```python
from build123d import *

# Parameters (mm, degrees)
SKETCH1_W               = 1500
SKETCH1_H               = 500
BOSS_EXTRUDE1_DEPTH     = 80
FILLET2_R               = 10
CUT_EXTRUDE2_START      = 80
SKETCH7_W               = 720
SKETCH7_H               = 439.016917436
CUT_EXTRUDE2_DEPTH      = 2
CUT_EXTRUDE1_START      = 78
SKETCH5_W               = 66
SKETCH5_H               = 45
CUT_EXTRUDE1_DEPTH      = 10
CUT_EXTRUDE3_START      = 80
SKETCH8_R               = 5
CUT_EXTRUDE3_DEPTH      = 875.606821013
CUT_EXTRUDE4_DEPTH      = 100
CUT_EXTRUDE4_DEPTH_BACK = 100
SKETCH9_W               = 720
SKETCH9_H               = 40
SKETCH11_R              = 10
CUT_EXTRUDE5_DEPTH      = 250


with BuildPart() as part:
    # Sketch1 → Boss-Extrude1 (new body)
    with BuildSketch(Plane(origin=(0, 0, 0), x_dir=(1, 0, 0), z_dir=(0, 1, 0))):
        Rectangle(SKETCH1_W, SKETCH1_H)
    extrude(amount=BOSS_EXTRUDE1_DEPTH)

    # Fillet2
    fillet2_edges = [part.edges().sort_by_distance(p)[0] for p in [
        (-750, 80, 0),
        (0, 80, 250),
        (750, 80, 0),
        (0, 80, -250),
    ]]
    fillet(fillet2_edges, radius=FILLET2_R)

    # Sketch7 → Cut-Extrude2 (cut)
    with BuildSketch(Plane(origin=(0, 0, 0), x_dir=(1, 0, 0), z_dir=(0, 1, 0)).offset(CUT_EXTRUDE2_START)):
        with Locations((0, 157.008458718)):
            Rectangle(SKETCH7_W, SKETCH7_H)
    extrude(amount=-CUT_EXTRUDE2_DEPTH, mode=Mode.SUBTRACT)

    # Sketch5 → Cut-Extrude1 (cut)
    with BuildSketch(Plane(origin=(0, 0, 0), x_dir=(1, 0, 0), z_dir=(0, 1, 0)).offset(CUT_EXTRUDE1_START)):
        with BuildLine():
            Line((-340, 52.5), (340, 52.5))
            ThreePointArc((340, 52.5), (347.071067812, 49.571067812), (350, 42.5))
            Line((350, 42.5), (350, -42.5))
            ThreePointArc((350, -42.5), (347.071067812, -49.571067812), (340, -52.5))
            Line((340, -52.5), (-340, -52.5))
            ThreePointArc((-340, -52.5), (-347.071067812, -49.571067812), (-350, -42.5))
            Line((-350, -42.5), (-350, 42.5))
            ThreePointArc((-350, 42.5), (-347.071067812, 49.571067812), (-340, 52.5))
        make_face()
        with BuildLine():
            Line((-340, 47.5), (-279, 47.5))
            Line((-279, 47.5), (-279, 7.071067812))
            ThreePointArc((-279, 7.071067812), (-281.803300859, 5.303300859), (-283.571067812, 2.5))
            Line((-283.571067812, 2.5), (-345, 2.5))
            Line((-345, 2.5), (-345, 42.5))
            ThreePointArc((-345, 42.5), (-343.535533906, 46.035533906), (-340, 47.5))
        make_face(mode=Mode.SUBTRACT)
        with BuildLine():
            Line((-340, -47.5), (-279, -47.5))
            Line((-279, -47.5), (-279, -7.071067812))
            ThreePointArc((-279, -7.071067812), (-281.803300859, -5.303300859), (-283.571067812, -2.5))
            Line((-283.571067812, -2.5), (-345, -2.5))
            Line((-345, -2.5), (-345, -42.5))
            ThreePointArc((-345, -42.5), (-343.535533906, -46.035533906), (-340, -47.5))
        make_face(mode=Mode.SUBTRACT)
        with BuildLine():
            Line((345, 42.5), (345, 2.5))
            Line((345, 2.5), (293.571067812, 2.5))
            ThreePointArc((293.571067812, 2.5), (291.803300859, 5.303300859), (289, 7.071067812))
            Line((289, 7.071067812), (289, 47.5))
            Line((289, 47.5), (340, 47.5))
            ThreePointArc((340, 47.5), (343.535533906, 46.035533906), (345, 42.5))
        make_face(mode=Mode.SUBTRACT)
        with Locations((-175, -25)):
            Rectangle(SKETCH5_W, SKETCH5_H, mode=Mode.SUBTRACT)
        with BuildLine():
            Line((0, 47.5), (0, 7.071067812))
            ThreePointArc((0, 7.071067812), (-2.803300859, 5.303300859), (-4.571067812, 2.5))
            Line((-4.571067812, 2.5), (-66, 2.5))
            Line((-66, 2.5), (-66, 47.5))
            Line((-66, 47.5), (0, 47.5))
        make_face(mode=Mode.SUBTRACT)
        with BuildLine():
            Line((5, 47.5), (5, 7.071067812))
            ThreePointArc((5, 7.071067812), (7.803300859, 5.303300859), (9.571067812, 2.5))
            Line((9.571067812, 2.5), (71, 2.5))
            Line((71, 2.5), (71, 47.5))
            Line((71, 47.5), (5, 47.5))
        make_face(mode=Mode.SUBTRACT)
        with Locations((-104, 25)):
            Rectangle(SKETCH5_W, SKETCH5_H, mode=Mode.SUBTRACT)
        with Locations((109, 25)):
            Rectangle(SKETCH5_W, SKETCH5_H, mode=Mode.SUBTRACT)
        with Locations((180, 25)):
            Rectangle(SKETCH5_W, SKETCH5_H, mode=Mode.SUBTRACT)
        with BuildLine():
            Line((218, 47.5), (218, 2.5))
            Line((218, 2.5), (279.428932188, 2.5))
            ThreePointArc((279.428932188, 2.5), (281.196699141, 5.303300859), (284, 7.071067812))
            Line((284, 7.071067812), (284, 47.5))
            Line((284, 47.5), (218, 47.5))
        make_face(mode=Mode.SUBTRACT)
        with Locations((-175, 25)):
            Rectangle(SKETCH5_W, SKETCH5_H, mode=Mode.SUBTRACT)
        with BuildLine():
            Line((-213, 47.5), (-213, 2.5))
            Line((-213, 2.5), (-269.428932188, 2.5))
            ThreePointArc((-269.428932188, 2.5), (-271.196699141, 5.303300859), (-274, 7.071067812))
            Line((-274, 7.071067812), (-274, 47.5))
            Line((-274, 47.5), (-213, 47.5))
        make_face(mode=Mode.SUBTRACT)
        with BuildLine():
            Line((-274, -7.071067812), (-274, -47.5))
            Line((-274, -47.5), (-213, -47.5))
            Line((-213, -47.5), (-213, -2.5))
            Line((-213, -2.5), (-269.428932188, -2.5))
            ThreePointArc((-269.428932188, -2.5), (-271.196699141, -5.303300859), (-274, -7.071067812))
        make_face(mode=Mode.SUBTRACT)
        with Locations((-104, -25)):
            Rectangle(SKETCH5_W, SKETCH5_H, mode=Mode.SUBTRACT)
        with BuildLine():
            Line((-66, -2.5), (-4.571067812, -2.5))
            ThreePointArc((-4.571067812, -2.5), (-2.803300859, -5.303300859), (0, -7.071067812))
            Line((0, -7.071067812), (0, -47.5))
            Line((0, -47.5), (-66, -47.5))
            Line((-66, -47.5), (-66, -2.5))
        make_face(mode=Mode.SUBTRACT)
        with BuildLine():
            Line((5, -7.071067812), (5, -47.5))
            Line((5, -47.5), (71, -47.5))
            Line((71, -47.5), (71, -2.5))
            Line((71, -2.5), (9.571067812, -2.5))
            ThreePointArc((9.571067812, -2.5), (7.803300859, -5.303300859), (5, -7.071067812))
        make_face(mode=Mode.SUBTRACT)
        with Locations((109, -25)):
            Rectangle(SKETCH5_W, SKETCH5_H, mode=Mode.SUBTRACT)
        with Locations((180, -25)):
            Rectangle(SKETCH5_W, SKETCH5_H, mode=Mode.SUBTRACT)
        with BuildLine():
            Line((218, -2.5), (218, -47.5))
            Line((218, -47.5), (284, -47.5))
            Line((284, -47.5), (284, -7.071067812))
            ThreePointArc((284, -7.071067812), (281.196699141, -5.303300859), (279.428932188, -2.5))
            Line((279.428932188, -2.5), (218, -2.5))
        make_face(mode=Mode.SUBTRACT)
        with BuildLine():
            Line((289, -7.071067812), (289, -47.5))
            Line((289, -47.5), (340, -47.5))
            ThreePointArc((340, -47.5), (343.535533906, -46.035533906), (345, -42.5))
            Line((345, -42.5), (345, -2.5))
            Line((345, -2.5), (293.571067812, -2.5))
            ThreePointArc((293.571067812, -2.5), (291.803300859, -5.303300859), (289, -7.071067812))
        make_face(mode=Mode.SUBTRACT)
    extrude(amount=-CUT_EXTRUDE1_DEPTH, mode=Mode.SUBTRACT)

    # Sketch8 → Cut-Extrude3 (cut, through all)
    with BuildSketch(Plane(origin=(0, 0, 0), x_dir=(1, 0, 0), z_dir=(0, 1, 0)).offset(CUT_EXTRUDE3_START)):
        with Locations(Location((-276.5, 0, 0), (0, 0, 270))):
            Circle(SKETCH8_R)
        with Locations(Location((2.5, 0, 0), (0, 0, 270))):
            Circle(SKETCH8_R)
        with Locations(Location((286.5, 0, 0), (0, 0, 270))):
            Circle(SKETCH8_R)
    extrude(amount=-CUT_EXTRUDE3_DEPTH, mode=Mode.SUBTRACT)

    # Sketch9 → Cut-Extrude4 (cut, two sides: drawn at the far end of the back side and taken through both)
    with BuildSketch(Plane.XY.offset(-CUT_EXTRUDE4_DEPTH_BACK)):
        with Locations((0, 20)):
            Rectangle(SKETCH9_W, SKETCH9_H)
    extrude(amount=CUT_EXTRUDE4_DEPTH + CUT_EXTRUDE4_DEPTH_BACK, mode=Mode.SUBTRACT)

    # Sketch11 → Cut-Extrude5 (cut)
    with BuildSketch(Plane.XY):
        with Locations(Location((0, 17.5, 0), (0, 0, 180))):
            Circle(SKETCH11_R)
    extrude(amount=CUT_EXTRUDE5_DEPTH, mode=Mode.SUBTRACT)


solid = part.part
```
For this review, take the finished solid that the model builds, in its own axes (mm). A direction names the side the tool comes from. Round coordinates to 2 decimals unless told otherwise and drop trailing zeros.
1) Machinability: for faces 1 (the face through (-175, 78, -25)), 2 (the face through (360, 20, -1)), 3 (the face through (-10, 80, 103)), which of the approach directions +Z, -Z, +X, -X, +Y, -Y give a long, thin tool a straight path to every point of the face, cutting with its end or side? Answer none if there is none.
Answer below:
face 1: -Z, +Y
face 2: -Y
face 3: +Z, -Z, +X, -X, +Y
2) For line 1 along X through (y, z) = (54.75, 0); line 2 along Z through (x, y) = (332.5, 68.5); line 3 along Z through (x, y) = (-307.5, 6), list the stretches that pass through material, from the lowest coordinate up.
Answer below:
line 1: x = -750 to -281.5, -271.5 to -2.5, 7.5 to 281.5, 291.5 to 750
line 2: z = -250 to -52.5, -47.5 to -2.5, 2.5 to 47.5, 52.5 to 250
line 3: z = -250 to -100, 100 to 250
3) Mouldability with a two-part tool opening along X and no side actions: class faces 4 (the face through (750, 35, 3)), 5 (the face through (-33, 78, 25)), 6 (the face through (-10, 35, -250)) as +X half, -X half, draft (parallel to the pull), parting line (faces both ways), or undercut.
Answer below:
face 4: +X half
face 5: undercut
face 6: draft
4) Insertion check: pin 1 Ø3 at (y, z) = (72.5, -30) entering from -X; pin 2 Ø22.5 at (x, z) = (26, 29) entering from +Y; pin 3 Ø5 at (y, z) = (75, -21) entering from +X; pin 4 Ø11 at (y, z) = (70.5, 34) entering from +X. Each pin has a flat end and moves straight along its axis. Give the tip position at first contact, or say it passes through.
Answer below:
pin 1: stops at x = -749.95
pin 2: stops at y = 78
pin 3: stops at x = 749.68
pin 4: stops at x = 750
